Geometry: final body of the model. Coordinates: model frame, mm. A direction names the side the tool comes from. Round coordinates to 2 decimals unless told otherwise and drop trailing zeros. Order: outer loops, then holes, each group sorted by start corner. A loop starts at its lowest first (then second) coordinate and runs counter-clockwise, first axis right, second up. Notation, with made-up numbers: M 32.5,54 L 48.5,54 A15 cw 48.5,61 Z; hole C 25.25,-8.5 d10. An arc over 180 degrees is marked long. Return JSON: item names as keys, results as strings. Group by question number.
Q1. Ray query, probe 1 along Z at (x, y) = (0.25, -11.5); probe 2 along Y at (x, z) = (0.5, -26); probe 3 along Y at (x, z) = (4.5, -8). Return the intervals inside material, ascending.
Q2. Cut plane A-A on z = -27.5. Output: boundary loops of the cut face in (x, y).
Q3. Mould query, pull axis Z, two halves, no side actions, for faces 6 (the face through (0, -70, 0)), 7 (the face through (-0.65, -60.14, -25.43)), 8 (the face through (-2.5, -34.5, 30)). Classes: released by +Z, released by -Z, zero draft, split by the parting line, or undercut.
Q4. Cut plane D-D on x = 2. Output: boundary loops of the cut face in (y, z), and give its area (3 significant figures).
Q5. Access query for faces 1 (the face through (0, -20, 23)), 2 (the face through (5, -35, -3)), 3 (the face through (-2.934, -33.048, -27.57)), 4 (the face through (3, -35, 27.5)), 5 (the face through (-0.65, -60.14, 19.57)). Directions: +Z, -Z, +X, -X, +Y, -Y. A direction counts if a zero-diameter tool reaches every point of the face in a straight line with its end or side. Return the directions, or none.
Q6. Contact query for flat-ended pins moving along their axis: pin 1 (3.5 mm diameter, centred on x = 0, z = -22.5, fed in from +Y); pin 2 (1.5 mm diameter, centred on x = 3, y = -43, fed in from +Z); pin 3 (3.5 mm diameter, centred on y = -25, z = -27.5, fed in from -X); pin 4 (2.5 mm diameter, centred on y = -39.5, z = 30.5, fed in from +X). Output: stop coordinate, or through.
Q7. Cut plane B-B on y = -35. Output: boundary loops of the cut face in (x, z), and give its area (4 significant figures).
Q8. Cut plane C-C on y = -25. Output: boundary loops of the cut face in (x, z).
```python
from build123d import *

# Parameters (mm, degrees)
F1_DEPTH  = 70
F3_R      = 2
F4_DEPTH  = 25
F6_R      = 3
F7_DEPTH  = 20
F8_R      = 3
F9_DEPTH  = 20
F10_R     = 3
F11_DEPTH = 20
F12_R     = 3
F13_DEPTH = 20
F2_R      = 2
F14_DEPTH = 10
F15_DEPTH = 25


with BuildPart() as f1:
    # F0 (on Front) → F1 (new body)
    with BuildSketch(Plane.XZ):
        Polygon((-5, 27.5), (-5, -32.5), (5, -32.5), (5, 27.5), (0, 27.5), (0, 32.5), align=None)
    extrude(amount=F1_DEPTH)

    # F3 (on face) → F4 (cut)
    with BuildSketch(Plane.YZ.offset(5)):
        with Locations((-45, -27.5)):
            Circle(F3_R)
        with Locations((-45, -7.5)):
            Circle(F3_R)
        with Locations((-25, -7.5)):
            Circle(F3_R)
        with Locations((-25, -27.5)):
            Circle(F3_R)
    extrude(amount=-F4_DEPTH, mode=Mode.SUBTRACT)

    # F6 (on face) → F7 (cut)
    with BuildSketch(Plane(origin=(0, 0, 0), x_dir=(-1, 0, 0), z_dir=(0, 1, 0))):
        with Locations((0, -22.5)):
            Circle(F6_R)
    extrude(amount=-F7_DEPTH, mode=Mode.SUBTRACT)

    # F8 (on face) → F9 (cut)
    with BuildSketch(Plane.XZ.offset(70)):
        with Locations((0, 22.5)):
            Circle(F8_R)
    extrude(amount=-F9_DEPTH, mode=Mode.SUBTRACT)

    # F10 (on face) → F11 (cut)
    with BuildSketch(Plane.XZ.offset(70)):
        with Locations((0, -22.5)):
            Circle(F10_R)
    extrude(amount=-F11_DEPTH, mode=Mode.SUBTRACT)

    # F12 (on face) → F13 (cut)
    with BuildSketch(Plane(origin=(0, 0, 0), x_dir=(-1, 0, 0), z_dir=(0, 1, 0))):
        with Locations((0, 22.5)):
            Circle(F12_R)
    extrude(amount=-F13_DEPTH, mode=Mode.SUBTRACT)

    # F2 (on face) → F14 (cut)
    with BuildSketch(Plane(origin=(0, 0, -32.5), x_dir=(1, 0, 0), z_dir=(0, 0, -1))):
        with Locations((-2.5, 35)):
            Circle(F2_R)
    extrude(amount=-F14_DEPTH, mode=Mode.SUBTRACT)

    # F3 (on face) → F15 (cut)
    with BuildSketch(Plane.YZ.offset(5)):
        with Locations((-45, -27.5)):
            Circle(F3_R)
        with Locations((-45, -7.5)):
            Circle(F3_R)
        with Locations((-25, -7.5)):
            Circle(F3_R)
        with Locations((-25, -27.5)):
            Circle(F3_R)
    extrude(amount=-F15_DEPTH, mode=Mode.SUBTRACT)


solid = f1.part
```
Result sheet:
{
 "1": {"probe 1": "z = -32.5 to -25.49, -19.51 to 19.51, 25.49 to 27.5", "probe 2": "y = -70 to -46.32, -43.68 to -26.32, -23.68 to 0", "probe 3": "y = -70 to -46.94, -43.06 to -26.94, -23.06 to 0"},
 "2": {"outline": "M -5,-70 L 5,-70 L 5,-47 L -5,-47 Z; M -5,-43 L 5,-43 L 5,-27 L -5,-27 Z; M -5,-23 L 5,-23 L 5,0 L -5,0 Z; hole C -2.5,-35 d4"},
 "3": {"face 6": "zero draft", "face 7": "undercut", "face 8": "released by +Z"},
 "4": {"outline": "M -70,-32.5 L 0,-32.5 L 0,-24.74 L -20,-24.74 L -20,-20.26 L 0,-20.26 L 0,20.26 L -20,20.26 L -20,24.74 L 0,24.74 L 0,27.5 L -70,27.5 L -70,24.74 L -50,24.74 L -50,20.26 L -70,20.26 L -70,-20.26 L -50,-20.26 L -50,-24.74 L -70,-24.74 Z; hole C -45,-27.5 d4; hole C -45,-7.5 d4; hole C -25,-27.5 d4; hole C -25,-7.5 d4", "area": "3,790 mm²"},
 "5": {"face 1": "+Y", "face 2": "+Z, -Z, +X, +Y, -Y", "face 3": "-Z", "face 4": "+Z, +X, +Y, -Y", "face 5": "-Y"},
 "6": {"pin 1": "stops at y = -20", "pin 2": "stops at z = 27.5", "pin 3": "passes through", "pin 4": "stops at x = 0"},
 "7": {"outline": "M -5,-32.5 L -4.5,-32.5 L -4.5,-22.5 L -0.5,-22.5 L -0.5,-32.5 L 5,-32.5 L 5,27.5 L 0,27.5 L 0,32.5 L -5,27.5 Z", "area": "572.5 mm²"},
 "8": {"outline": "M -5,-32.5 L 5,-32.5 L 5,-29.5 L -5,-29.5 Z; M -5,-25.5 L 5,-25.5 L 5,-9.5 L -5,-9.5 Z; M -5,-5.5 L 5,-5.5 L 5,27.5 L 0,27.5 L 0,32.5 L -5,27.5 Z"}
}
